Check sheet for the drawn part. Datum: minimum x, y, z corner. Units: mm. A direction names the side the tool comes from. Coordinates: 2 decimals unless noted, no trailing zeros. Write each loop counter-clockwise with the first axis right and the second up, starting at its lowest first coordinate (ties: lowest second). Pieces come first, ordered by that corner, then holes. Notation, with made-up numbers: (46.5, 89.25) - (86.5, 89.25) arc R14 ccw to (86.5, 98.25) - close; hole circle Ø2 at (29.5, 88). An arc over 180 degrees is marked (long way). Use one line per item in the form item = value. Start each with the question number.
1. Cross-section at D-D on x = 97. Record the boundary of the cut face in (y, z) (1 decimal), then the cut area to 3 significant figures.
2. Cross-section at A-A on z = 2.75. Record the boundary of the cut face in (x, y), then the cut area to 3 significant figures.
3. Scan lines: line 1 along X through (y, z) = (64, 18.5); line 2 along X through (y, z) = (34, 4.75); line 3 along X through (y, z) = (11, 18.5). Record each from-to range of solid material in increasing order.
4. Tool access check on the marked faces 4 and 5. Record the directions out of +Z, -Z, +X, -X, +Y, -Y that give a thin tool (end or side, any length) a straight path to the whole face; none if there is none.
5. Draft check along X on the marked faces 1, 2 and 3. Enter one of: +X half, -X half, draft (parallel to the pull), parting line (faces both ways), or undercut.
6. Cross-section at C-C on y = 39. Record the boundary of the cut face in (x, z), then the cut area to 4 significant figures.
7. Go/stop test with flat-tipped pins: pin 1 Ø5 at (x, z) = (111.5, 4) entering from -Y; pin 2 Ø2.5 at (x, z) = (180, 8) entering from +Y; pin 3 Ø2.5 at (x, z) = (3, 15) entering from +Y. Record where each tip stops, or that it passes through.
8. Cross-section at B-B on x = 77.5. Record the boundary of the cut face in (y, z) (1 decimal), then the cut area to 3 significant figures.
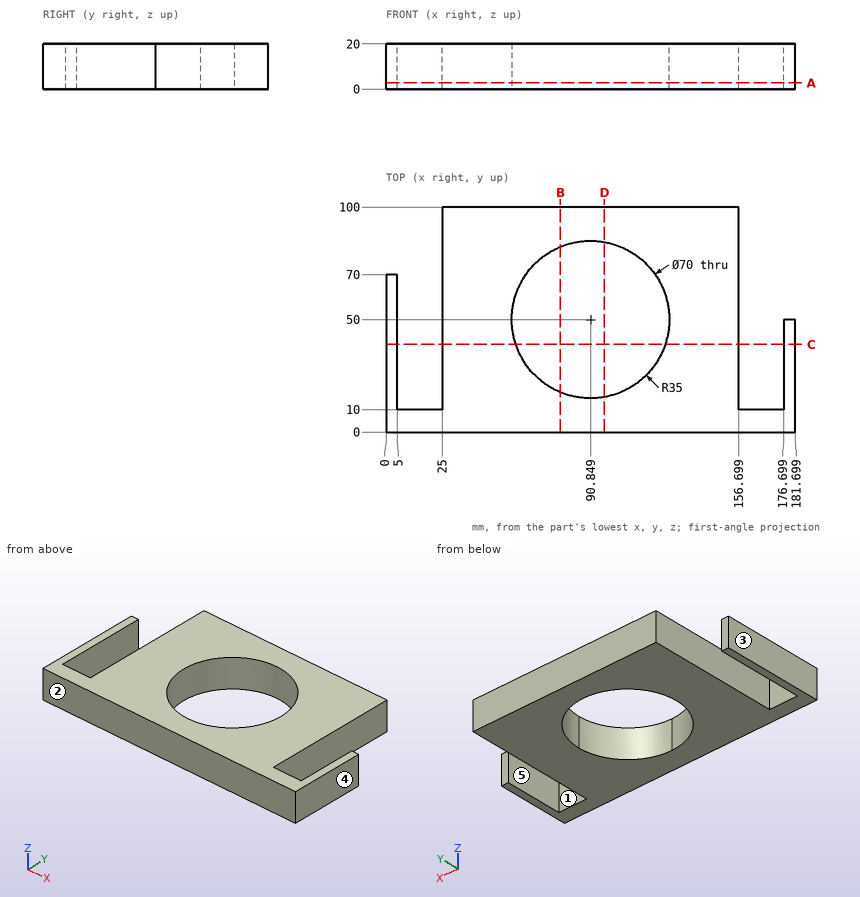
Final values:
q1.outline = (0, 0) - (15.5, 0) - (15.5, 20) - (0, 20) - close; (84.5, 0) - (100, 0) - (100, 20) - (84.5, 20) - close
q1.area = 622 mm²
q2.outline = (0, 0) - (181.7, 0) - (181.7, 50) - (176.7, 50) - (176.7, 10) - (156.7, 10) - (156.7, 100) - (25, 100) - (25, 10) - (5, 10) - (5, 70) - (0, 70) - close; hole (90.85, 15) arc R35 ccw to (125.85, 50) arc R35 ccw (long way) to start
q2.area = 10,300 mm²
q3.line_1 = 0 to 5, 25 to 58.77, 122.93 to 156.7
q3.line_2 = 0 to 5, 25 to 59.72, 121.98 to 156.7, 176.7 to 181.7
q3.line_3 = 0 to 5, 25 to 156.7, 176.7 to 181.7
q4.face_4 = +Z, -Z, +X, +Y, -Y
q4.face_5 = +Z, -Z, +Y
q5.face_1 = undercut
q5.face_2 = draft
q5.face_3 = -X half
q6.outline = (0, 0) - (5, 0) - (5, 20) - (0, 20) - close; (25, 0) - (57.62, 0) - (57.62, 20) - (25, 20) - close; (124.08, 0) - (156.7, 0) - (156.7, 20) - (124.08, 20) - close; (176.7, 0) - (181.7, 0) - (181.7, 20) - (176.7, 20) - close
q6.area = 1,505 mm²
q7.pin_1 = 0
q7.pin_2 = 50
q7.pin_3 = 70
q8.outline = (0, 0) - (17.6, 0) - (17.6, 20) - (0, 20) - close; (82.4, 0) - (100, 0) - (100, 20) - (82.4, 20) - close
q8.area = 706 mm²
